Autodesk Inventor part; units mm, degrees
ref_plane "YZ Plane" through (0, 0, 0) normal (1, 0, 0) x (0, 1, 0)
ref_plane "XZ Plane" through (0, 0, 0) normal (0, 1, 0) x (-1, 0, 0)
ref_plane "XY Plane" through (0, 0, 0) normal (0, 0, 1) x (1, 0, 0)
sketch "Sketch1" plane through (0, 0, 0) normal (0, 0, 1) x (1, 0, 0)
  line L0 (40, -40) -> (-40, -40)
  line L1 (-40, -40) -> (-40, 40)
  line L2 (-40, 40) -> (40, 40)
  line L3 (40, 40) -> (40, -40)
  line L4 (40, -40) -> (-40, 40) construction
  line L5 (-40, -40) -> (40, 40) construction
  line L6 (-37, -37) -> (37, -37)
  line L7 (37, -37) -> (37, 37)
  line L8 (37, 37) -> (-37, 37)
  line L9 (-37, 37) -> (-37, -37)
  point P0 (0, 0)
  dimension "d0" = 80
  dimension "d1" = 80
  dimension "d2" = 3
extrude "Extrusion1" add sketch "Sketch1" along normal blind 172.4121
sketch "Sketch2" plane through (0, 0, 0) normal (1, 0, 0) x (0, 1, 0)
  line L0 (40, 0) -> (-40, 0)
  line L1 (-40, 0) -> (-40, 172.4121)
  line L2 (40, 172.4121) -> (-40, 172.4121)
  line L3 (40, 0) -> (40, 172.4121)
  line L4 (40, 172.4121) -> (-40, 148.3319)
  point P0 (0, 0)
  dimension "d5" = 16.752
extrude "Extrusion2" cut sketch "Sketch2" along normal through all both and the other way through all contours L4 L1 L2
equation "\"d3\" = Lenth"
equation "\"d5\" = Leg_cut_angle"
equation "\"Lenth\" = Leg_hight"
properties part number "ANP 1484 leg tube"
Read the model definition and answer for the solid it produces. Units are mm, in the model's axes. A direction names the side the tool comes from. Round coordinates to 2 decimals unless told otherwise and drop trailing zeros. Write each loop counter-clockwise with the first axis right and the second up, starting at its lowest first coordinate (ties: lowest second). Pieces come first, ordered by that corner, then holes.
Q1. Find section A-A on x = 22.5. Determine the outline of the cut face in (y, z).
Values:
outline: (-40, 0) - (-37, 0) - (-37, 149.23) - (-40, 148.33) - close; (37, 0) - (40, 0) - (40, 172.41) - (37, 171.51) - close
Q2. Straight lines are drawn through the part: line 1 (X direction, y = 31, z = 44); line 2 (Y direction, x = 7.5, z = 162.5). For each, find the intervals that lie inside material, in ascending order.
Values:
line 1: x = -40 to -37, 37 to 40
line 2: y = 37 to 40
Q3. Find section C-C on y = -13. Determine the outline of the cut face in (x, z), and give its area (3 significant figures).
Values:
outline: (-40, 0) - (-37, 0) - (-37, 156.46) - (-40, 156.46) - close; (37, 0) - (40, 0) - (40, 156.46) - (37, 156.46) - close
area: 939 mm2
Q4. The mould has two halves that part along Y. Classify faces 1 (the face through (-37, 1, 85)), 2 (the face through (-3, -38, 0)), 3 (the face through (38.33, 3.15, 161.32)): released by +Y, released by -Y, zero draft, split by the parting line, or undercut.
Values:
face 1: undercut
face 2: zero draft
face 3: released by -Y
Q5. A tool of negligible diameter and unlimited length cuts with its end or side. For faces 4 (the face through (-40, -1, 85)), 5 (the face through (1, 37, 85)), from which of +Z, -Z, +X, -X, +Y, -Y can it reach the whole face along a straight path? Write none if from no direction.
Values:
face 4: +Z, -Z, -X, +Y, -Y
face 5: +Z, -Z
Q6. Find section B-B on z = 30.5. Determine the outline of the cut face in (x, y).
Values:
outline: (-40, -40) - (40, -40) - (40, 40) - (-40, 40) - close; hole (-37, -37) - (37, -37) - (37, 37) - (-37, 37) - close
